Geometry: final body of the model. Coordinates: model frame, mm. A direction names the side the tool comes from. Give positions to 0.01 mm unless a question says otherwise; leave off trailing zeros. Write each loop counter-clockwise with the first axis right and the second up, starting at its lowest first coordinate (ties: lowest second). Pieces come first, ordered by that corner, then holes.
Q1. Section B-B (z = 7.75). Return the cut outline in (x, y), plus the area to 3 significant figures.
Q2. Reachability of faces 4 (the flat face through (20, -75, 5)), 5 (the flat face through (0, -67, 0)), 6 (the flat face through (-20, -75, 5)) from +Z, -Z, +X, -X, +Y, -Y: full face, straight path, thin tool, end or side. Return the list, or none.
Q3. Mould query, pull axis X, two halves, no side actions, for faces 1 (the flat face through (-25, -90, 5)), 2 (the conical face through (-1.599, -3.075, 6.746)), 3 (the flat face through (0, 10, 0)). Classes: +X half, -X half, draft (parallel to the pull), parting line (faces both ways), or undercut.
Q4. Section D-D (x = 8). Return the cut outline in (y, z).
Q5. Section A-A (x = 0). Return the cut outline in (y, z), plus the area to 3 significant figures.
Q6. Pin query (flat end, axial travel): pin 1 Ø3 at (x, z) = (-19, 5.5) entering from +Y; pin 2 Ø5 at (x, z) = (-4.5, -5) entering from -Y; pin 3 Ø3 at (x, y) = (7.5, -51) entering from -Z. Return the tip coordinate at first contact, or that it passes through.
Q7. Line query: line 1 (Y direction, x = 0, z = 3.25); line 2 (X direction, y = 0, z = 3); line 3 (X direction, y = -95, z = 2.5). Output: solid intervals per line, ascending.
Q8. Section C-C (y = 0). Return the cut outline in (x, z).
from build123d import *

# Parameters (mm, degrees)
F1_DEPTH       = 15
F2_W           = 50
F2_H           = 10
F3_DEPTH       = 30
F5_D           = 6.6
F5_DEPTH       = 20
F5_CSINK_D     = 13.44
F5_CSINK_ANGLE = 90
F5_TIP         = 1.9828400428
F7_D           = 6.6
F7_DEPTH       = 10
F7_CSINK_D     = 13.44
F7_CSINK_ANGLE = 90
F7_TIP         = 1.9828400428


with BuildPart() as f1:
    # F0 (on Right) → F1 (new body, symmetric)
    with BuildSketch(Plane.YZ):
        Polygon((10, -10), (10, 10), (-10, 10), (-75, 10), (-75, 0), (-10, 0), (-10, -10), align=None)
    extrude(amount=F1_DEPTH, both=True)

    # F2 (on face) → F3 (join)
    with BuildSketch(Plane.XZ.offset(75)):
        with Locations((0, 5)):
            Rectangle(F2_W, F2_H)
    extrude(amount=F3_DEPTH)

    # F5
    with Locations(Plane.XY.offset(10)):
        with Locations((0, 0)):
            CounterSinkHole(F5_D / 2, F5_CSINK_D / 2, depth=F5_DEPTH, counter_sink_angle=F5_CSINK_ANGLE)
            with Locations((0, 0, -(F5_DEPTH + F5_TIP / 2))):  # 118° drill point
                Cone(0, F5_D / 2, F5_TIP, mode=Mode.SUBTRACT)

    # F7
    with Locations(Plane.XY.offset(10)):
        with Locations((0, -95)):
            CounterSinkHole(F7_D / 2, F7_CSINK_D / 2, depth=F7_DEPTH, counter_sink_angle=F7_CSINK_ANGLE)
            with Locations((0, 0, -(F7_DEPTH + F7_TIP / 2))):  # 118° drill point
                Cone(0, F7_D / 2, F7_TIP, mode=Mode.SUBTRACT)


solid = f1.part
Computed:
1. outline: (-25, -105) - (25, -105) - (25, -75) - (15, -75) - (15, 10) - (-15, 10) - (-15, -75) - (-25, -75) - close; hole circle Ø8.94 at (0, -95); hole circle Ø8.94 at (0, 0)
1. area: 3,920 mm2
2. face 4: +Z, -Z, +X, +Y
2. face 5: -Z, +X, -X, -Y
2. face 6: +Z, -Z, -X, +Y
3. face 1: -X half
3. face 2: undercut
3. face 3: draft
4. outline: (-105, 0) - (-10, 0) - (-10, -10) - (10, -10) - (10, 10) - (-105, 10) - close
5. outline: (-105, 0) - (-98.3, 0) - (-98.3, 6.58) - (-101.72, 10) - (-105, 10) - close; (-91.7, 0) - (-10, 0) - (-10, -10) - (-3.3, -10) - (-3.3, 6.58) - (-6.72, 10) - (-88.28, 10) - (-91.7, 6.58) - close; (3.3, -10) - (10, -10) - (10, 10) - (6.72, 10) - (3.3, 6.58) - close
5. area: 1,130 mm2
6. pin 1: stops at y = -75
6. pin 2: stops at y = -10
6. pin 3: stops at z = 0
7. line 1: y = -105 to -98.3, -91.7 to -3.3, 3.3 to 10
7. line 2: x = -15 to -3.3, 3.3 to 15
7. line 3: x = -25 to -3.3, 3.3 to 25
8. outline: (-15, -10) - (-3.3, -10) - (-3.3, 6.58) - (-6.72, 10) - (-15, 10) - close; (3.3, -10) - (15, -10) - (15, 10) - (6.72, 10) - (3.3, 6.58) - close
